from build123d import *

# Parameters (mm, degrees)
SCHNITT_LINEAR_AUSTRAGEN1_DEPTH = 2.056247308


with BuildPart() as part:
    # Skizze1 → Rotation1 (revolve)
    with BuildSketch(Plane.XY):
        with BuildLine():
            Line((-3, -0.986868648), (-1.5, -0.986868648))
            Line((-1.5, -0.986868648), (-1.5, -7.722161257))
            Line((-1.5, -7.722161257), (0, -7.722161257))
            Line((0, -7.722161257), (0, 1.056247208))
            add(Edge.make_bspline(
                [(-3, 0.013131352), (-1.65504596, 1.020141519), (0, 1.056247208)],
                knots=[0, 0, 0, 0.690587557, 0.690587557, 0.690587557], degree=2))
            Line((-3, 0.013131352), (-3, -0.986868648))
        make_face()
    revolve(axis=Axis((0, 54.476945253, 0), (0, -1, 0)))

    # Skizze2 → Schnitt-Linear austragen1 (cut, through all)
    with BuildSketch(Plane(origin=(0, 0, 0), x_dir=(1, 0, 0), z_dir=(0, 1, 0))):
        Polygon((-0.4, 3.573663987), (0.4, 3.573663987), (0.4, 0.395605851), (1.5, 0.395605851), (1.5, -0.43040926), (0.4, -0.43040926), (0.4, -3.41246381), (-0.4, -3.41246381), (-0.4, -0.43040926), (-1.5, -0.43040926), (-1.5, 0.395605851), (-0.4, 0.395605851), align=None)
    extrude(amount=SCHNITT_LINEAR_AUSTRAGEN1_DEPTH, mode=Mode.SUBTRACT)


solid = part.part
Source: CAD feature listing. Evaluate the final solid. Frame: model axes, mm. A direction names the side the tool comes from. Round coordinates to 2 decimals unless told otherwise and drop trailing zeros. Order: outer loops, then holes, each group sorted by start corner. A loop starts at its lowest first (then second) coordinate and runs counter-clockwise, first axis right, second up. Notation, with made-up numbers: (87, 79.25) - (114, 79.25) arc R34 cw to (114, 113.25) - close; hole circle Ø6 at (25, 88.25). An arc over 180 degrees is marked (long way). Use a Markdown table: item, result. Add a question column.
1. Line query: probe 1 along Y at (x, z) = (-0.75, 0.4); probe 2 along Y at (x, z) = (0, 2.1); probe 3 along X at (y, z) = (-6, 0.2). Output: solid intervals per line, ascending.
2. Section query A-A (x = 0). Return the cut outline in (y, z).
3. Set-up query: faces 1 (the flat face through (0, -7.722, 0)), 2 (the cylindrical face through (3, -0.5, -0.1)), 3 (the flat face through (-0.4, 0.4, -1.4)), 4 (the flat face through (-1.3, -0.987, 1.3)), 5 (the flat face through (-1, 0.5, -0.396)). Return all of +Z, -Z, +X, -X, +Y, -Y with unobstructed straight access to the full face (end or side cutting, diameter ignored); none if empty.
4. Section query B-B (y = -0.5). Return the cut outline in (x, z).
5. Mould query, pull axis Z, two halves, no side actions, for faces 6 (the cylindrical face through (1.5, -4.4, -0.07)), 7 (the flat face through (1.5, 0.4, 0)), 8 (the flat face through (0.4, 0.4, 1.4)). Classes: +Z half, -Z half, draft (parallel to the pull), parting line (faces both ways), or undercut.
6. Section query C-C (y = -2.25). Return the cut outline in (x, z), then the cut area to 3 significant figures.
7. First-contact query: pin 1 (2 mm diameter, centred on x = -1.5, y = -1, fed in from +Z); pin 2 (1.5 mm diameter, centred on x = 0.5, z = 1.5, fed in from +Y); pin 3 (0.5 mm diameter, centred on x = 1, y = 0.5, fed in from -Z). Flat tips, straight axial feed; report the tip coordinate or a pass-through.
Derived:
| question | item | result |
|---|---|---|
| 1 | probe 1 | -7.72 to 0 |
| 1 | probe 2 | -0.99 to 0 |
| 1 | probe 3 | -1.49 to 1.49 |
| 2 | outline | (-7.72, -1.5) - (-0.99, -1.5) - (-0.99, -3) - (0, -3) - (0, 3) - (-0.99, 3) - (-0.99, 1.5) - (-7.72, 1.5) - close |
| 3 | face 1 | +Z, -Z, +X, -X, -Y |
| 3 | face 2 | +Y, -Y |
| 3 | face 3 | +Z, -Z, +Y |
| 3 | face 4 | -Y |
| 3 | face 5 | +Y |
| 4 | outline | circle Ø6 at (0, 0) |
| 5 | face 6 | parting line |
| 5 | face 7 | undercut |
| 5 | face 8 | draft |
| 6 | outline | circle Ø3 at (0, 0) |
| 6 | area | 7.07 mm2 |
| 7 | pin 1 | z = 2.96 |
| 7 | pin 2 | y = 0.97 |
| 7 | pin 3 | z = -2.47 |
